Could you check a few things on this model? Use its own coordinates, in mm. Give positions to 0.01 mm unless a question says otherwise; leave off trailing zeros. Write each loop counter-clockwise with the first axis right and the second up, starting at its lowest first coordinate (ties: lowest second). Pieces come first, ordered by that corner, then holes. Notation, with made-up numbers: (35, 58) - (49, 58) arc R26 ccw to (49, 96) - close; hole circle Ø3 at (62.25, 24). An arc over 180 degrees is marked (long way). Use one line per item in the form item = value.
```python
from build123d import *

# Parameters (mm, degrees)
F3_DEPTH = 25


# Not quite as in the source:
# - the program builds the solid bodies; features that only make, move or delete a surface that nothing else refers to are left out


with BuildPart() as f3:
    # F2 (on Right) → F3 (new body)
    with BuildSketch(Plane.YZ):
        with BuildLine():
            ThreePointArc((-56.4248897135, 62.7899920644), (-56.4100056303, 63.0273500708), (-56.4050413852, 63.2651224732))
            ThreePointArc((-56.4050413852, 63.2651224732), (-62.1018148959, 68.9618959839), (-67.7985884065, 63.2651224732))
            Line((-67.7985884065, 63.2651224732), (-56.4248897135, 63.2651224732))
            Line((-56.4248897135, 63.2651224732), (-56.4248897135, 62.7899920644))
        make_face()
        with BuildLine():
            Line((-56.4628131563, 46.0544750094), (-67.7606649638, 46.0544750094))
            ThreePointArc((-67.7606649638, 46.0544750094), (-62.11173906, 40.4055491057), (-56.4628131563, 46.0544750094))
        make_face()
        with BuildLine():
            Line((-56.4248897135, 63.2651224732), (-67.7985884065, 63.2651224732))
            ThreePointArc((-67.7985884065, 63.2651224732), (-62.3395872983, 57.5733132076), (-56.4248897135, 62.7899920644))
            Line((-56.4248897135, 62.7899920644), (-56.4248897135, 63.2651224732))
        make_face()
        with BuildLine():
            ThreePointArc((-56.4248897135, 62.7899920644), (-62.3395872983, 57.5733132076), (-67.7985884065, 63.2651224732))
            Line((-67.7985884065, 63.2651224732), (-67.7985884065, 46.0544750094))
            Line((-67.7985884065, 46.0544750094), (-67.7606649638, 46.0544750094))
            ThreePointArc((-67.7606649638, 46.0544750094), (-62.11173906, 51.7034009132), (-56.4628131563, 46.0544750094))
            Line((-56.4628131563, 46.0544750094), (-56.4248897135, 46.0544750094))
            Line((-56.4248897135, 46.0544750094), (-56.4248897135, 62.7899920644))
        make_face()
        with BuildLine():
            ThreePointArc((-56.4628131563, 46.0544750094), (-62.11173906, 51.7034009132), (-67.7606649638, 46.0544750094))
            Line((-67.7606649638, 46.0544750094), (-56.4628131563, 46.0544750094))
        make_face()
    extrude(amount=F3_DEPTH)


solid = f3.part
```
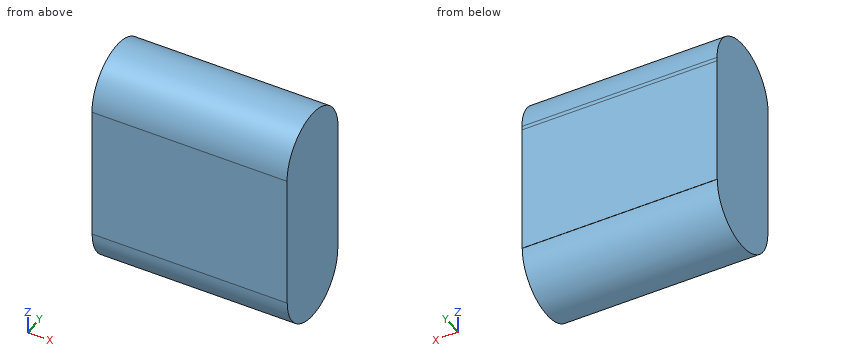
1. Imagine slicing it at C-C, the plane z = 45. List the corners of the cut face in (x, y) for me.
Response values:
outline = (0, -67.66) - (25, -67.66) - (25, -56.56) - (0, -56.56) - close
2. For pin 1 (1 mm diameter, centred on y = -65, z = 51.5, fed in from -X); pin 2 (3 mm diameter, centred on x = 10.5, y = -58, fed in from +Z); pin 3 (8.5 mm diameter, centred on x = 11.5, z = 58.5, fed in from +Y), each with a flat end and sliding along its axis, tell me the tip position at first contact or that it passes through.
Response values:
pin_1 = 0
pin_2 = 68.33
pin_3 = -56.42
3. Imagine slicing it at B-B, the plane y = -60.5. List the corners of the cut face in (x, z) for me.
Response values:
outline = (0, 40.64) - (25, 40.64) - (25, 68.73) - (0, 68.73) - close
4. If I drill on line 1 (Y direction, x = 20.5, z = 60); line 2 (Z direction, x = 15.5, y = -66.75); line 3 (Y direction, x = 15.75, z = 67.25), over which ranges is the centre line in solid material (lowest first)? Write a range as from..to.
Response values:
line_1 = -67.8..-56.42
line_2 = 42.83..66.56
line_3 = -66.17..-58.03
